```python
from build123d import *

# Parameters (mm, degrees)
SKETCH_W     = 76.2
SKETCH_H     = 25.4
SKETCH_R     = 4.7625
PAD_DEPTH    = 1.905
CHAMFER_SIZE = 1.000001
SKETCH001_W  = 12.7
SKETCH001_H  = 12.7
POCKET_DEPTH = 0.254
FILLET_R     = 1.27


with BuildPart() as part:
    # Sketch → Pad (new body)
    with BuildSketch(Plane.XY):
        Rectangle(SKETCH_W, SKETCH_H)
        Circle(SKETCH_R, mode=Mode.SUBTRACT)
        with Locations((-19.05, 0)):
            Circle(SKETCH_R, mode=Mode.SUBTRACT)
        with Locations((19.05, 0)):
            Circle(SKETCH_R, mode=Mode.SUBTRACT)
    extrude(amount=PAD_DEPTH)

    # Chamfer
    chamfer_edges = [part.edges().sort_by_distance(p)[0] for p in [
        (14.2875, 0, 0),
        (-4.7625, 0, 0),
        (-23.8125, 0, 0),
    ]]
    chamfer(chamfer_edges, length=CHAMFER_SIZE)

    # Sketch001 (on Face3 of Chamfer) → Pocket (cut)
    with BuildSketch(Plane.XY.offset(1.905)):
        Rectangle(SKETCH001_W, SKETCH001_H)
        with Locations((-19.05, 0)):
            Rectangle(SKETCH001_W, SKETCH001_H)
        with Locations((19.05, 0)):
            Rectangle(SKETCH001_W, SKETCH001_H)
    extrude(amount=-POCKET_DEPTH, mode=Mode.SUBTRACT)

    # Fillet
    fillet_edges = [part.edges().sort_by_distance(p)[0] for p in [
        (38.1, 12.7, 0.9525),
        (38.1, -12.7, 0.9525),
        (-38.1, 12.7, 0.9525),
        (-38.1, -12.7, 0.9525),
    ]]
    fillet(fillet_edges, radius=FILLET_R)


solid = part.part
```
Build history of the part. All positions in model axes, mm. A direction names the side the tool comes from. Round coordinates to 2 decimals unless told otherwise and drop trailing zeros.
1) 3-axis set-ups, long thin cutter, end or side, ignore diameter. For faces 5 (the flat face through (-1, 6, 0)), 6 (the flat face through (23, -3, 1.651)): which of +Z, -Z, +X, -X, +Y, -Y reach the whole face in a straight line?
2) Drill centre lines: probe 1 along X at (y, z) = (0, 1.4); probe 2 along X at (y, z) = (4, 1.75); probe 3 along Y at (x, z) = (-3, 1.85). Where is each one in solid material? Low to high.
3) Pin check, flat tips, straight feed: pin 1 (6.5 mm diameter, centred on x = -20.5, y = 1, fed in from +Z); pin 2 (5.5 mm diameter, centred on x = 19.05, y = 0, fed in from -Z). Stop position of each tip, or through.
4) Mould opens along X. For faces 1 (the flat face through (-1, 12.7, 1)), 2 (the flat face through (-15, 3, 1.651)), 3 (the flat face through (-38.1, 0, 1)), 4 (the flat face through (3, 4, 1.651)) say: +X half, -X half, draft (parallel to the pull), parting line (faces both ways), or undercut.
5) Band-saw the part on A-A, the plane y = 0. Give the number of separate pieces and of enclosed holes in the cut face, and give its area (3 significant figures).
Ans:
1. face 5: -Z, +X, -X, +Y, -Y
1. face 6: +Z
2. probe 1: x = -38.1 to -23.81, -14.29 to -4.76, 4.76 to 14.29, 23.81 to 38.1
2. probe 2: x = -38.1 to -25.4, -12.7 to -6.35, 6.35 to 12.7, 25.4 to 38.1
2. probe 3: y = -12.7 to -6.35, 6.35 to 12.7
3. pin 1: stops at z = 1.65
3. pin 2: passes through
4. face 1: draft
4. face 2: undercut
4. face 3: -X half
4. face 4: undercut
5. separate pieces: 4
5. enclosed holes: 0
5. area: 85.3 mm2
